Can you work these out from the model? Positions are in its coordinate system, mm. Face numbers are marked on the shaded views. Round coordinates to 2 decimals unless told otherwise and drop trailing zeros. Loops run counter-clockwise (first coordinate to the right, second up) from the corner with the lowest first, then second, coordinate; pieces in that order, holes last. Notation, with made-up numbers: M 82.25,25 L 116.25,25 A23 cw 116.25,56 Z; hole C 84.25,12 d9. An arc over 180 degrees is marked long. Use a Markdown table: item, result. Add a question column.
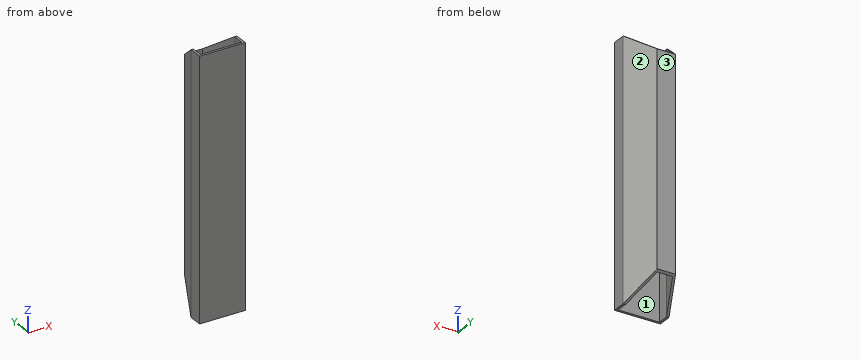
```python
from build123d import *

# Parameters (mm, degrees)
BOSS_EXTRUDE1_DEPTH = 112
CUT_EXTRUDE1_DEPTH  = 113
CUT_EXTRUDE2_DEPTH  = 21
CUT_EXTRUDE3_DEPTH  = 21


with BuildPart() as part:
    # Sketch1 → Boss-Extrude1 (new body)
    with BuildSketch(Plane.XY):
        Polygon((-4, 14), (4, 14), (10, 0), (10, -6), (-10, -6), (-10, 0), align=None)
    extrude(amount=BOSS_EXTRUDE1_DEPTH)

    # Sketch2 → Cut-Extrude1 (cut, through all)
    with BuildSketch(Plane.XY.offset(112)):
        Polygon((-3.340603842, 13), (-9, -0.205257702), (-9, -5), (9, -5), (9, -0.205257702), (3.340603842, 13), align=None)
    extrude(amount=-CUT_EXTRUDE1_DEPTH, mode=Mode.SUBTRACT)

    # Sketch4 → Cut-Extrude2 (cut, through all)
    with BuildSketch(Plane(origin=(10, 0, 0), x_dir=(0, 0, -1), z_dir=(1, 0, 0))):
        Polygon((-112, 14), (-102, 14), (-112, 0), align=None)
    extrude(amount=-CUT_EXTRUDE2_DEPTH, mode=Mode.SUBTRACT)

    # Sketch5 → Cut-Extrude3 (cut, through all)
    with BuildSketch(Plane.ZY.offset(10)):
        Polygon((0, 14), (10, 14), (0, 0), align=None)
    extrude(amount=-CUT_EXTRUDE3_DEPTH, mode=Mode.SUBTRACT)


solid = part.part
```
(1) I'm going to push flat-ended pins straight in: pin 1 (1.5 mm diameter, centred on x = 0, y = -3, fed in from -Z); pin 2 (3 mm diameter, centred on x = -7, z = 98, fed in from +Y); pin 3 (12 mm diameter, centred on y = 8, z = 61.5, fed in from +X); pin 4 (4 mm diameter, centred on x = -7.5, y = 7, fed in from +Z). Where does each tip first touch, or does it pass through?
(2) Suppose I cut it at A-A on y = -1.5. List the corners of the cut face in (x, z) for me.
(3) Suppose I cut it at B-B on z = 91.5. List the corners of the cut face in (x, y) for me.
(4) Thinking about a two-plate mould opening in X: for the marked faces 1, 2 and 3, which applies, released by +X, released by -X, zero draft, split by the parting line, or undercut?
(5) If I drill on probe 1 along X at (y, z) = (-2, 88.5); probe 2 along Y at (x, z) = (-1.5, 45.5); probe 3 along X at (y, z) = (9, 50), over which ranges is the centre line in solid material (lowest first)? Write a range as [from, to].
(6) Suppose I cut it at C-C on x = -0.75. List the corners of the cut face in (y, z) for me, and give its area (3 significant figures).
Results below:
| question | item | result |
|---|---|---|
| 1 | pin 1 | passes through |
| 1 | pin 2 | stops at y = 10.5 |
| 1 | pin 3 | stops at x = 9.14 |
| 1 | pin 4 | stops at z = 108.43 |
| 2 | outline | M -10,0 L -9,0 L -9,112 L -10,112 Z; M 9,0 L 10,0 L 10,112 L 9,112 Z |
| 3 | outline | M -10,-6 L 10,-6 L 10,0 L 4,14 L -4,14 L -10,0 Z; hole M -9,-5 L 9,-5 L 9,-0.21 L 3.34,13 L -3.34,13 L -9,-0.21 Z |
| 4 | face 1 | undercut |
| 4 | face 2 | released by +X |
| 4 | face 3 | zero draft |
| 5 | probe 1 | x = [-10, -9], [9, 10] |
| 5 | probe 2 | y = [-6, -5], [13, 14] |
| 5 | probe 3 | x = [-6.14, -5.05], [5.05, 6.14] |
| 6 | outline | M -6,0 L -5,0 L -5,112 L -6,112 Z; M 13,9.29 L 14,10 L 14,102 L 13,102.71 Z |
| 6 | area | 205 mm² |
